Autodesk Fusion 360 part; units mm, degrees
sketch "Sketch1" plane through (0, 0, 0) normal (0, 0, 1) x (1, 0, 0)
  line L0 (28.485, 84.19) -> (0, 84.19)
  line L1 (36.985, 0) -> (36.985, 75.69)
  line L2 (0, 0) -> (0, 84.19) construction
  line L3 (0, 0) -> (36.985, 0) construction
  arc A0 (36.985, 75.69) -> (28.485, 84.19) centre (28.485, 75.69) ccw
  line L4 (-28.485, 84.19) -> (0, 84.19)
  arc A1 (-28.485, 84.19) -> (-36.985, 75.69) centre (-28.485, 75.69) ccw
  line L5 (-36.985, 0) -> (-36.985, 75.69)
  line L6 (36.985, 0) -> (36.985, -75.69)
  arc A2 (28.485, -84.19) -> (36.985, -75.69) centre (28.485, -75.69) ccw
  line L7 (28.485, -84.19) -> (0, -84.19)
  line L8 (-28.485, -84.19) -> (0, -84.19)
  arc A3 (-36.985, -75.69) -> (-28.485, -84.19) centre (-28.485, -75.69) ccw
  line L9 (-36.985, 0) -> (-36.985, -75.69)
  line L10 (-36.985, 58.3417) -> (-37.985, 58.3417)
  line L11 (-37.985, 58.3417) -> (-37.985, 38.3417)
  line L12 (-37.985, 38.3417) -> (-36.985, 38.3417)
  line L13 (-36.985, 38.3417) -> (-36.985, 58.3417)
  line L14 (-37.985, 38.3417) -> (-36.985, 38.3417)
  line L15 (-36.985, 38.3417) -> (-36.985, 13.3417)
  line L16 (-36.985, 13.3417) -> (-37.985, 13.3417)
  line L17 (-37.985, 13.3417) -> (-37.985, 38.3417)
  line L18 (36.985, 55.0141) -> (37.985, 55.0141)
  line L19 (37.985, 55.0141) -> (37.985, 45.0141)
  line L20 (37.985, 45.0141) -> (36.985, 45.0141)
  line L21 (36.985, 45.0141) -> (36.985, 55.0141)
  dimension "d3" = 8.5
  dimension "d4" = 1
  dimension "d5" = 20
  dimension "d6" = 25
  dimension "d7" = 1
  dimension "d8" = 10
extrude "Extrude1" add sketch "Sketch1" along normal blind 9.69
fillet "Fillet1" radius 2 5 edges at (-36.985, -31.1741, 9.69) (-34.4954, -81.7004, 9.69) (0, -84.19, 9.69) (34.4954, -81.7004, 9.69) (36.985, -15.3379, 9.69)
CAD build for the part. Positions are in the model's coordinates, mm. A direction names the side the tool comes from. Round coordinates to 2 decimals unless told otherwise and drop trailing zeros. Write each loop counter-clockwise with the first axis right and the second up, starting at its lowest first coordinate (ties: lowest second). Pieces come first, ordered by that corner, then holes. Notation, with made-up numbers: (14, -18.5) -> (32, -18.5) arc R27 cw to (32, 3.5) -> close; hole circle Ø4 at (49.5, 24.5). An arc over 180 degrees is marked (long way). Answer in a Markdown table with one row per item. Add a question column.
Item 1: Drop flat-ended pins along their axis: pin 1 Ø3 at (y, z) = (63.5, 4) entering from -X (3 decimals); pin 2 Ø5 at (y, z) = (66.5, 7) entering from +X (3 decimals); pin 3 Ø0.5 at (x, z) = (-37.5, 5) entering from +Y; pin 4 Ø4 at (x, y) = (-28.5, -45.5) entering from -Z. Give the stop position or say it passes through.
Item 2: Saw through at C-C, the plane y = 69.5. Write the cut outline in (x, z) (3 decimals).
Item 3: Drill centre lines: line 1 (X direction, y = 32.5, z = 5.5) (3 decimals); line 2 (X direction, y = -56.5, z = 7.75); line 3 (Y direction, x = 13.5, z = 8). Where is each one in solid material? Low to high. Write a range as from..to.
Item 4: Mould opens along Z. For faces 1 (the face through (-1, 1, 0)), 2 (the face through (-1, 2, 9.69)), 3 (the face through (0, -84.19, 4)) say: pulls with the +Z half, pulls with the -Z half, needs draft (parallel to the pull), parting line crosses it, or undercut.
Item 5: Saw through at B-B, the plane y = -3. Write the cut outline in (x, z) (3 decimals), then the cut area to 3 significant figures.
Item 6: Which spindle directions (+Z, -Z, +X, -X, +Y, -Y) get a long thin tool onto all of the face, cutting with end or side? Do faces 4 (the face through (36.985, -16, 4)), 5 (the face through (-36.985, 67, 5)), 6 (the face through (36.985, 65, 5)), 7 (the face through (-36.985, -31, 4)), 8 (the face through (37.985, 50, 5)). Say none if no direction does.
Item 7: Saw through at A-A, the plane z = 4.75. Write the cut outline in (x, y) (3 decimals).
Findings below:
| question | item | result |
|---|---|---|
| 1 | pin 1 | stops at x = -36.985 |
| 1 | pin 2 | stops at x = 36.985 |
| 1 | pin 3 | stops at y = 58.34 |
| 1 | pin 4 | stops at z = 0 |
| 2 | outline | (-36.985, 0) -> (36.985, 0) -> (36.985, 9.69) -> (-36.985, 9.69) -> close |
| 3 | line 1 | x = -37.985..36.985 |
| 3 | line 2 | x = -36.98..36.98 |
| 3 | line 3 | y = -84.17..84.19 |
| 4 | face 1 | pulls with the -Z half |
| 4 | face 2 | pulls with the +Z half |
| 4 | face 3 | needs draft |
| 5 | outline | (-36.985, 0) -> (36.985, 0) -> (36.985, 7.69) arc R2 ccw to (34.985, 9.69) -> (-34.985, 9.69) arc R2 ccw to (-36.985, 7.69) -> close |
| 5 | area | 715 mm^2 |
| 6 | face 4 | +Z, -Z, +X, -Y |
| 6 | face 5 | +Z, -Z, -X, +Y |
| 6 | face 6 | +Z, -Z, +X, +Y |
| 6 | face 7 | +Z, -Z, -X, -Y |
| 6 | face 8 | +Z, -Z, +X, +Y, -Y |
| 7 | outline | (-37.985, 13.342) -> (-36.985, 13.342) -> (-36.985, -75.69) arc R8.5 ccw to (-28.485, -84.19) -> (28.485, -84.19) arc R8.5 ccw to (36.985, -75.69) -> (36.985, 45.014) -> (37.985, 45.014) -> (37.985, 55.014) -> (36.985, 55.014) -> (36.985, 75.69) arc R8.5 ccw to (28.485, 84.19) -> (-28.485, 84.19) arc R8.5 ccw to (-36.985, 75.69) -> (-36.985, 58.342) -> (-37.985, 58.342) -> close |
